```python
from build123d import *

# Parameters (mm, degrees)
MODEL_R                 = 5
MODEL_W                 = 3
MODEL_H                 = 18.163611367
MODEL_H_2               = 18.163611368
SALIENTE_EXTRUIR1_DEPTH = 3


with BuildPart() as part:
    # Model → Saliente-Extruir1 (new body)
    with BuildSketch(Plane.XY):
        with BuildLine():
            Line((110.507104, 49.029117707), (-17.27548715, 49.029117707))
            ThreePointArc((-17.27548715, 49.029117707), (-17.98412567, 48.739950134), (-18.280736421, 48.034394679))
            Line((-18.280736421, 48.034394679), (-18.313224497, 41.861702909))
            ThreePointArc((-18.313224497, 41.861702909), (-18.609835248, 41.156147454), (-19.318473769, 40.866979881))
            Line((-19.318473769, 40.866979881), (-35.492896, 40.856340442))
            ThreePointArc((-35.492896, 40.856340442), (-36.200002781, 40.563447224), (-36.492896, 39.856340442))
            Line((-36.492896, 39.856340442), (-36.492896, -24.470882293))
            ThreePointArc((-36.492896, -24.470882293), (-36.200002781, -25.177989074), (-35.492896, -25.470882293))
            Line((-35.492896, -25.470882293), (-19.492896, -25.470882293))
            ThreePointArc((-19.492896, -25.470882293), (-18.785789219, -25.763775512), (-18.492896, -26.470882293))
            Line((-18.492896, -26.470882293), (-18.492896, -32.643659558))
            ThreePointArc((-18.492896, -32.643659558), (-18.200002781, -33.350766339), (-17.492896, -33.643659558))
            Line((-17.492896, -33.643659558), (26.507104, -33.643659558))
            Line((26.507104, -33.643659558), (32.507104, -33.643659558))
            Line((32.507104, -33.643659558), (65.191293724, -33.643659558))
            Line((65.191293724, -33.643659558), (110.507104, -33.643659558))
            ThreePointArc((110.507104, -33.643659558), (111.214210781, -33.350766339), (111.507104, -32.643659558))
            Line((111.507104, -32.643659558), (111.507104, 48.029117707))
            ThreePointArc((111.507104, 48.029117707), (111.214210781, 48.736224488), (110.507104, 49.029117707))
        make_face()
        with Locations((7.707104, 7.592729075)):
            Circle(MODEL_R, mode=Mode.SUBTRACT)
        Polygon((10.507104, 18.329117707), (4.507104, 18.329117707), (4.507104, 13.829117707), (-3.492896, 13.829117707), (-3.492896, 18.329117707), (-9.492896, 18.329117707), (-9.492896, 29.329117707), (-3.492896, 29.329117707), (-3.492896, 33.829117707), (4.507104, 33.829117707), (4.507104, 29.329117707), (10.507104, 29.329117707), align=None, mode=Mode.SUBTRACT)
        Polygon((10.507104, -3.143659558), (4.507104, -3.143659558), (4.507104, 1.356340442), (-3.492896, 1.356340442), (-3.492896, -3.143659558), (-9.492896, -3.143659558), (-9.492896, -14.143659558), (-3.492896, -14.143659558), (-3.492896, -18.643659558), (4.507104, -18.643659558), (4.507104, -14.143659558), (10.507104, -14.143659558), align=None, mode=Mode.SUBTRACT)
        with Locations((-26.792896, 21.774534758)):
            Rectangle(MODEL_W, MODEL_H, mode=Mode.SUBTRACT)
        with Locations((-26.792896, -6.389076609)):
            Rectangle(MODEL_W, MODEL_H_2, mode=Mode.SUBTRACT)
    extrude(amount=SALIENTE_EXTRUIR1_DEPTH)


solid = part.part
```
Geometry check sheet. Reference: the model listing, model coordinates, mm. A direction names the side the tool comes from. Coordinates: 2 decimals unless noted, no trailing zeros. Answer in a Markdown table with one row per item. Add a question column.
1. Section check A-A (z = 1.95). Give the number of separate pieces and of enclosed holes in the cut face, plus the area to 3 significant figures.
2. Draft check along Y on faces 3 (the face through (36, 8, 3)), 4 (the face through (-3.493, 16, 1)), 5 (the face through (-28, -25.471, 1)). Enter one of: +Y half, -Y half, draft (parallel to the pull), parting line (faces both ways), or undercut.
3. Gauge pin test, flat ends, axial feed: pin 1 Ø0.9 at (x, z) = (-26, 2) entering from -Y; pin 2 Ø1.5 at (x, z) = (-26.5, 1.5) entering from +Y. Record the tip position at first contact, or that the pin passes through.
4. Material ranges on L1, parallel to X at y = 25.5, z = 0.1; L2, parallel to X at y = 14, z = 0.65; L3, parallel to Y at x = -1.5, z = 2, recorded low to high. Write a range as [from, to].
5. Access from +Z, -Z, +X, -X, +Y, -Y to the whole of each face (thin tool, end or side, straight path). Record for faces 1 (the face through (48, 49.029, 1)), 2 (the face through (0, -18.644, 1)).
Data:
| question | item | result |
|---|---|---|
| 1 | separate pieces | 1 |
| 1 | enclosed holes | 5 |
| 1 | area | 11,200 mm² |
| 2 | face 3 | draft |
| 2 | face 4 | undercut |
| 2 | face 5 | -Y half |
| 3 | pin 1 | stops at y = -25.47 |
| 3 | pin 2 | stops at y = 40.86 |
| 4 | L1 | x = [-36.49, -28.29], [-25.29, -9.49], [10.51, 111.51] |
| 4 | L2 | x = [-36.49, -28.29], [-25.29, -3.49], [4.51, 111.51] |
| 4 | L3 | y = [-33.64, -18.64], [1.36, 13.83], [33.83, 49.03] |
| 5 | face 1 | +Z, -Z, +X, -X, +Y |
| 5 | face 2 | +Z, -Z |
